Input: part model. Units: mm. Frame: model coordinates. Round coordinates to 2 decimals unless told otherwise and drop trailing zeros. Loops run counter-clockwise (first coordinate to the right, second up) from the corner with the lowest first, then second, coordinate; pieces in that order, holes last. Notation, with made-up numbers: (-1, 43.5) -> (7, 43.5) arc R22 cw to (7, 78.5) -> close; hole circle Ø7 at (77.5, 37.5). An arc over 180 degrees is marked (long way). One line per question, with ' | ' between items. Start each with the question number.
Q1. Material intervals for L1, parallel to Z at x = -3, y = 0.35; L2, parallel to X at y = 3.6, z = 7.5; L3, parallel to X at y = 3.55, z = 3.25, sorted ascending.
Q2. Contact query for flat-ended pins moving along their axis: P1, Ø1.5, axis at y = 3, z = -7, coming from the +X side; P2, Ø1, axis at y = 2, z = -2.5, coming from the -X side; P3, Ø2, axis at x = 8, y = 2.5, coming from the +Z side. Output: stop coordinate, or through.
Q3. Cut plane A-A on y = 0.95. Return loops of the section in (x, z), and give its area (3 significant figures).
Q4. Mould query, pull axis Z, two halves, no side actions, for faces 1 (the face through (10.89, 0.09, 0.03)), 2 (the face through (9.051, 1.972, 5.324)), 3 (the face through (4.57, 1.972, -7.167)). Classes: pulls with the +Z half, pulls with the -Z half, needs draft (parallel to the pull), parting line crosses it, or undercut.
from build123d import *

# Parameters (mm, degrees)
SKETCH_1_R          = 8.5
EXTRUDE_1_DEPTH     = 4
SKETCH_2_OUTSIDE_W  = 76.028
SKETCH_2_OUTSIDE_H  = 72.78
SKETCH_2_OUTSIDE_R  = 10.5
CUT_EXTRUDE_1_DEPTH = 5
CUT_EXTRUDE_1_TAPER = 77
SKETCH_3_OUTSIDE_W  = 76.028
SKETCH_3_OUTSIDE_H  = 72.78
SKETCH_3_OUTSIDE_R  = 10.5
CUT_EXTRUDE_2_DEPTH = 5
CUT_EXTRUDE_2_TAPER = 77


with BuildPart() as part:
    # Эскиз1 → Бобышка-Вытянуть1 (new body)
    with BuildSketch(Plane(origin=(0, 0, 0), x_dir=(1, 0, 0), z_dir=(0, 1, 0))):
        Polygon((12.124355653, 0), (6.062177826, 10.5), (-6.062177826, 10.5), (-12.124355653, 0), (-6.062177826, -10.5), (6.062177826, -10.5), align=None)
        Circle(SKETCH_1_R, mode=Mode.SUBTRACT)
    extrude(amount=EXTRUDE_1_DEPTH)

    # Эскиз2 outside → Вырез-Вытянуть1 (cut, through all)
    with BuildSketch(Plane(origin=(0, 4, 0), x_dir=(1, 0, 0), z_dir=(0, 1, 0))):
        Rectangle(SKETCH_2_OUTSIDE_W, SKETCH_2_OUTSIDE_H)
        Circle(SKETCH_2_OUTSIDE_R, mode=Mode.SUBTRACT)
    extrude(amount=-CUT_EXTRUDE_1_DEPTH, taper=CUT_EXTRUDE_1_TAPER, mode=Mode.SUBTRACT)

    # Эскиз3 outside → Вырез-Вытянуть2 (cut, through all)
    with BuildSketch(Plane.XZ):
        Rectangle(SKETCH_3_OUTSIDE_W, SKETCH_3_OUTSIDE_H)
        Circle(SKETCH_3_OUTSIDE_R, mode=Mode.SUBTRACT)
    extrude(amount=-CUT_EXTRUDE_2_DEPTH, taper=CUT_EXTRUDE_2_TAPER, mode=Mode.SUBTRACT)


solid = part.part
Results:
1) L1: -10.5 to -7.95, 7.95 to 10.5 | L2: -7.79 to -4, 4 to 7.79 | L3: -10.25 to -7.85, 7.85 to 10.25
2) P1: x = 8.52 | P2: x = -10.97 | P3: z = 8.88
3) outline: (-12.12, 0) -> (-6.06, -10.5) -> (6.06, -10.5) -> (12.12, 0) -> (6.06, 10.5) -> (-6.06, 10.5) -> close; hole circle Ø17 at (0, 0) | area: 155 mm^2
4) face 1: parting line crosses it | face 2: pulls with the +Z half | face 3: undercut
